Design review of the part shown in the three views and the two pictorial views. Dimensions are in mm from the part's minimum x, y and z. A direction names the side the tool comes from. Coordinates: 2 decimals unless noted, no trailing zeros. Loops run counter-clockwise (first coordinate to the right, second up) from the corner with the lowest first, then second, coordinate; pieces in that order, holes last. Notation, with made-up numbers: (20.5, 86) - (67.5, 86) arc R4 cw to (67.5, 93) - close; hole circle Ø2 at (0.25, -17). An arc over 180 degrees is marked (long way). One line per item, written item: value. Start each with the question number.
1. To check wall thickness, follow line 1 (X direction, y = 46, z = 41); line 2 (Z direction, x = 18.5, y = 78). State the ranges of each line that lie inside material, in increasing order. Write a range as from..to.
2. Insertion check: pin 1 (24 mm diameter, centred on y = 39.5, z = 27, fed in from -X); pin 2 (8 mm diameter, centred on x = 25, z = 55.5, fed in from +Y); pin 3 (5 mm diameter, centred on x = 51, y = 53, fed in from -Z); pin 4 (12 mm diameter, centred on x = 24, z = 20, fed in from -Y). Each pin has a flat end and moves straight along its axis. Give the tip position at first contact, or say it passes through.
3. The part is to be moulded in two halves that separate along Z. For the marked faces 5, 6 and 7, say which applies: released by +Z, released by -Z, zero draft, split by the parting line, or undercut.
4. Take a section at B-B, the plane x = 54.5. State the section outline as (y, z) points, and give its area (3 significant figures).
5. Take a section at A-A, the plane y = 13. State the section outline as (x, z) points.
6. For the marked faces 1, 2, 3 and 4, list the 3-axis set-ups (+Z, -Z, +X, -X, +Y, -Y) from which the entire face can be reached by the end or side of a thin tool; tool diameter is ignored.
7. Take a section at C-C, the plane z = 45. State the section outline as (x, y) points, and give its area (4 significant figures).
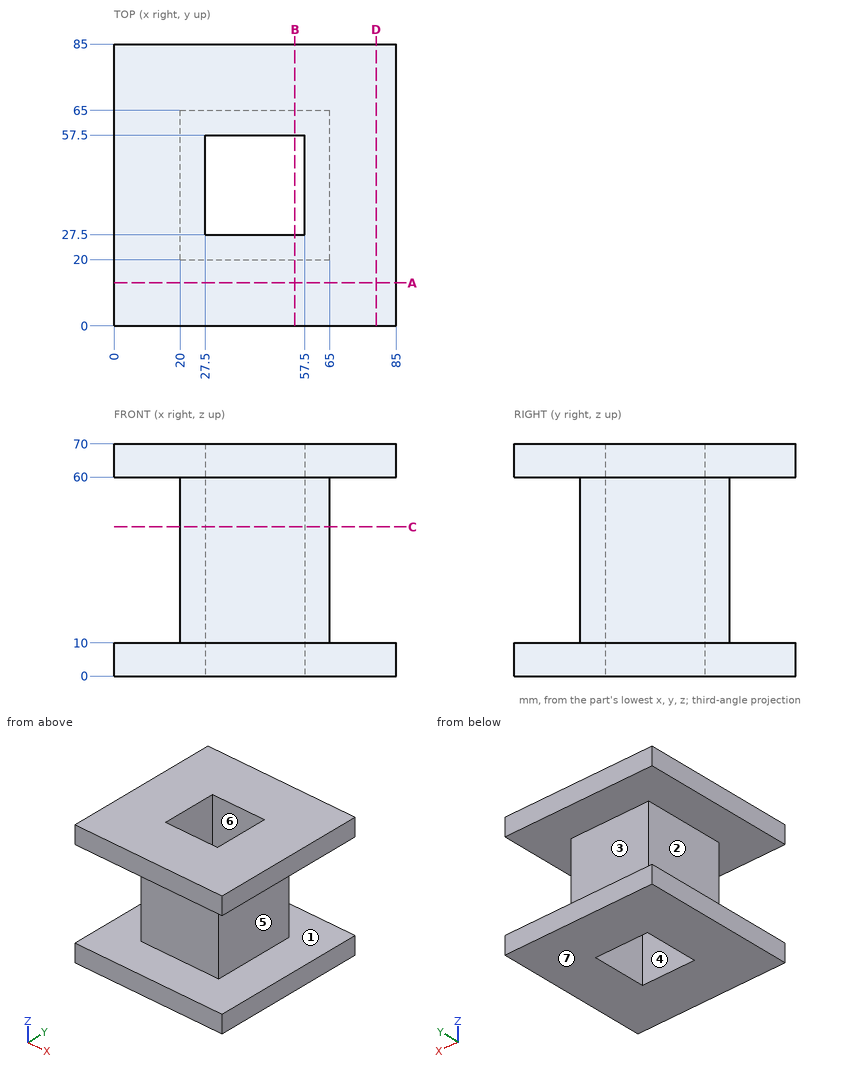
Solutions:
1. line 1: 20..27.5, 57.5..65
1. line 2: 0..10, 60..70
2. pin 1: x = 20
2. pin 2: y = 65
2. pin 3: through
2. pin 4: y = 20
3. face 5: undercut
3. face 6: zero draft
3. face 7: released by -Z
4. outline: (0, 0) - (27.5, 0) - (27.5, 70) - (0, 70) - (0, 60) - (20, 60) - (20, 10) - (0, 10) - close; (57.5, 0) - (85, 0) - (85, 10) - (65, 10) - (65, 60) - (85, 60) - (85, 70) - (57.5, 70) - close
4. area: 1,850 mm2
5. outline: (0, 0) - (85, 0) - (85, 10) - (0, 10) - close; (0, 60) - (85, 60) - (85, 70) - (0, 70) - close
6. face 1: none
6. face 2: -X, +Y, -Y
6. face 3: +X, -X, +Y
6. face 4: +Z, -Z
7. outline: (20, 20) - (65, 20) - (65, 65) - (20, 65) - close; hole (27.5, 27.5) - (57.5, 27.5) - (57.5, 57.5) - (27.5, 57.5) - close
7. area: 1,125 mm2
